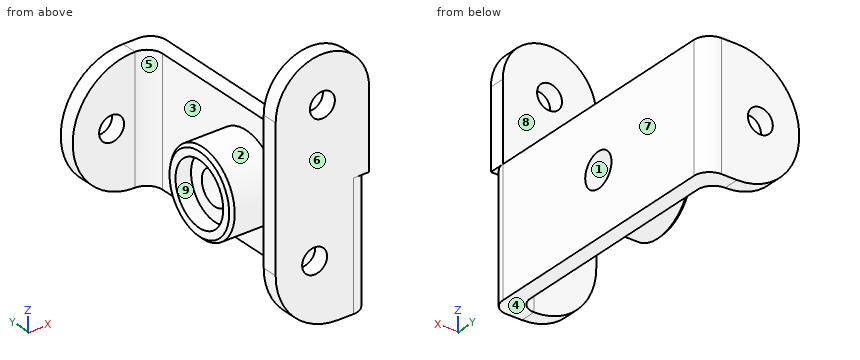
```python
from build123d import *

# Parameters (mm, degrees)
BOSS_EXTRUDE2_DEPTH             = 20
SKETCH2_R                       = 13.5
SKETCH2_R_2                     = 5.5
BOSS_EXTRUDE3_DEPTH             = 15
CUT_EXTRUDE1_DEPTH              = 56.226805086
CUT_EXTRUDE1_DEPTH_BACK         = 56.226805086
SKETCH2_3_R                     = 5.5
CHAMFER1_SIZE                   = 1
SKETCH3_R                       = 4
CUT_EXTRUDE2_DEPTH              = 10
FILLET2_RADIUS                  = 20
FILLET2_LENGTH                  = 5
FILLET3_RADIUS                  = 20
FILLET3_LENGTH                  = 5
SKETCH4_R                       = 4
CUT_EXTRUDE3_DEPTH              = 10
BOSS_EXTRUDE4_DEPTH             = 40
BOSS_EXTRUDE4_DIRECTION_2_REACH = 69.268
SKETCH7_R                       = 4
CUT_EXTRUDE4_DEPTH              = 30
FILLET5_RADIUS                  = 15
FILLET5_LENGTH                  = 5
SKETCH8_R                       = 10
CUT_EXTRUDE5_DEPTH              = 5


with BuildPart() as part:
    # Sketch1 → Boss-Extrude2 (new, symmetric)
    with BuildSketch(Plane.XY):
        with BuildLine():
            Line((0, 45), (25, 45))
            ThreePointArc((25, 45), (28.535533906, 43.535533906), (30, 40))
            Line((30, 40), (30, -40))
            ThreePointArc((30, -40), (28.535533906, -43.535533906), (25, -45))
            Line((25, -45), (0, -45))
            Line((0, -45), (0, -40))
            Line((0, -40), (20, -40))
            ThreePointArc((20, -40), (23.535533906, -38.535533906), (25, -35))
            Line((25, -35), (25, 35))
            ThreePointArc((25, 35), (23.535533906, 38.535533906), (20, 40))
            Line((20, 40), (0, 40))
            Line((0, 40), (0, 45))
        make_face()
    extrude(amount=BOSS_EXTRUDE2_DEPTH, both=True)

    # Sketch2 → Boss-Extrude3 (add)
    # profile 1 of 2: a face of its own
    with BuildSketch(Plane.ZY.offset(-25)):
        with Locations(Location((0, 0, 0), (0, 0, 180))):
            Circle(SKETCH2_R)
        Circle(SKETCH2_R_2, mode=Mode.SUBTRACT)
    # profile 2 of 2: a face of its own
    with BuildSketch(Plane.ZY.offset(-25)):
        Circle(SKETCH2_R_2)
    extrude(amount=BOSS_EXTRUDE3_DEPTH)

    # Sketch2<3> → Cut-Extrude1 (cut, two sides: drawn at the far end of the back side and taken through both)
    with BuildSketch(Plane.ZY.offset(-25).offset(-CUT_EXTRUDE1_DEPTH_BACK)):
        with Locations(Location((0, 0, 0), (0, 0, 270))):
            Circle(SKETCH2_3_R)
    extrude(amount=CUT_EXTRUDE1_DEPTH + CUT_EXTRUDE1_DEPTH_BACK, mode=Mode.SUBTRACT)

    # Chamfer1
    chamfer1_edges = [part.edges().sort_by_distance(p)[0] for p in [
        (10, 0, 13.5),
    ]]
    chamfer(chamfer1_edges, length=CHAMFER1_SIZE)

    # Sketch3 → Cut-Extrude2 (cut)
    with BuildSketch(Plane(origin=(0, 45, 0), x_dir=(1, 0, 0), z_dir=(0, 1, 0))):
        with Locations(Location((12.5, 0, 0), (0, 0, 180))):
            Circle(SKETCH3_R)
    extrude(amount=-CUT_EXTRUDE2_DEPTH, mode=Mode.SUBTRACT)

    # Fillet2: full round fillet: the end face becomes a half cylinder, R = half its width
    fillet2_face = Plane((0, 42.5, 0), x_dir=(0, -1, 0), z_dir=(-1, 0, 0))  # on the end face: x along it, z out of the body
    fillet2_slab = fillet2_face.offset(-FILLET2_RADIUS / 2) * Box(FILLET2_LENGTH, 2 * FILLET2_RADIUS, FILLET2_RADIUS, mode=Mode.PRIVATE)  # the body's end, R deep
    fillet2_round = Plane((20, 42.5, 0), x_dir=(-1, 0, 0), z_dir=(0, -1, 0)) * Cylinder(FILLET2_RADIUS, FILLET2_LENGTH, mode=Mode.PRIVATE)  # its axis R under the face
    add(fillet2_slab - fillet2_round, mode=Mode.SUBTRACT)

    # Fillet3: full round fillet: the end face becomes a half cylinder, R = half its width
    fillet3_face = Plane((0, -42.5, 0), x_dir=(0, -1, 0), z_dir=(-1, 0, 0))  # on the end face: x along it, z out of the body
    fillet3_slab = fillet3_face.offset(-FILLET3_RADIUS / 2) * Box(FILLET3_LENGTH, 2 * FILLET3_RADIUS, FILLET3_RADIUS, mode=Mode.PRIVATE)  # the body's end, R deep
    fillet3_round = Plane((20, -42.5, 0), x_dir=(-1, 0, 0), z_dir=(0, -1, 0)) * Cylinder(FILLET3_RADIUS, FILLET3_LENGTH, mode=Mode.PRIVATE)  # its axis R under the face
    add(fillet3_slab - fillet3_round, mode=Mode.SUBTRACT)

    # Sketch4 → Cut-Extrude3 (cut)
    with BuildSketch(Plane(origin=(0, -40, 0), x_dir=(1, 0, 0), z_dir=(0, 1, 0))):
        with Locations(Location((12.5, 0, 0), (0, 0, 180))):
            Circle(SKETCH4_R)
    extrude(amount=-CUT_EXTRUDE3_DEPTH, mode=Mode.SUBTRACT)

    # Sketch6 → Boss-Extrude4 (add)
    with BuildSketch(Plane.XY.offset(20)):
        Polygon((0, -40), (0, -45), (30, -45), (30, -40), (20, -40), align=None)
    extrude(amount=BOSS_EXTRUDE4_DEPTH)

    # Sketch6 → Boss-Extrude4 direction 2 (add, up to next)
    with BuildSketch(Plane.XY.offset(20), mode=Mode.PRIVATE) as boss_extrude4_direction_2_sk1:
        Polygon((0, -40), (0, -45), (30, -45), (30, -40), (20, -40), align=None)
    boss_extrude4_direction_2_tool1 = extrude(boss_extrude4_direction_2_sk1.sketch, amount=-BOSS_EXTRUDE4_DIRECTION_2_REACH, mode=Mode.PRIVATE) - part.part
    add(boss_extrude4_direction_2_tool1.solids().sort_by_distance((15, -42.5, 20))[0])

    # Sketch7 → Cut-Extrude4 (cut)
    with BuildSketch(Plane(origin=(0, -40, 0), x_dir=(1, 0, 0), z_dir=(0, 1, 0))):
        with Locations(Location((15, -45, 0), (0, 0, 180))):
            Circle(SKETCH7_R)
    extrude(amount=-CUT_EXTRUDE4_DEPTH, mode=Mode.SUBTRACT)

    # Fillet5: full round fillet: the end face becomes a half cylinder, R = half its width
    fillet5_face = Plane((15, -42.5, 60), x_dir=(0, -1, 0), z_dir=(0, 0, 1))  # on the end face: x along it, z out of the body
    fillet5_slab = fillet5_face.offset(-FILLET5_RADIUS / 2) * Box(FILLET5_LENGTH, 2 * FILLET5_RADIUS, FILLET5_RADIUS, mode=Mode.PRIVATE)  # the body's end, R deep
    fillet5_round = Plane((15, -42.5, 45), x_dir=(0, 0, 1), z_dir=(0, -1, 0)) * Cylinder(FILLET5_RADIUS, FILLET5_LENGTH, mode=Mode.PRIVATE)  # its axis R under the face
    add(fillet5_slab - fillet5_round, mode=Mode.SUBTRACT)

    # Sketch8 → Cut-Extrude5 (cut)
    with BuildSketch(Plane.ZY.offset(-10)):
        with Locations(Location((0, 0, 0), (0, 0, 270))):
            Circle(SKETCH8_R)
    extrude(amount=-CUT_EXTRUDE5_DEPTH, mode=Mode.SUBTRACT)


solid = part.part
```
Geometry: final body of the model. Coordinates: model frame, mm. Face numbers are marked on the shaded views. A direction names the side the tool comes from. Give positions to 0.01 mm unless a question says otherwise; leave off trailing zeros. Write each loop counter-clockwise with the first axis right and the second up, starting at its lowest first coordinate (ties: lowest second). Pieces come first, ordered by that corner, then holes.
1. Pin query (flat end, axial travel): P1, Ø1, axis at x = 8.5, z = 38.5, coming from the +Y side; P2, Ø14.5, axis at y = 0, z = 0, coming from the -X side; P3, Ø12, axis at x = 16, y = -23.5, coming from the +Z side; P4, Ø20, axis at y = -0.5, z = -1.5, coming from the -X side. Return the tip coordinate at first contact, or that it passes through.
2. Section query D-D, the plane x = 26. Return loops of the section in (y, z).
3. Section query C-C, the plane z = 47.5. Return loops of the section in (x, y).
4. Reachability of the marked faces 5, 6, 7, 8 and 9 from +Z, -Z, +X, -X, +Y, -Y: full face, straight path, thin tool, end or side. Return the list, or none.
5. Section query A-A, the plane y = 0. Return loops of the section in (x, z).
6. Line query: probe 1 along Y at (x, z) = (6, 13); probe 2 along Y at (x, z) = (19, 6); probe 3 along Z at (x, y) = (12.5, -42). Output: solid intervals per line, ascending.
7. Draft query along Z for the marked faces 1, 2, 3 and 4. Return one class per face: released by +Z, released by -Z, zero draft, split by the parting line, or undercut.
8. Section query B-B, the plane x = 12.5. Return loops of the section in (y, z).
Computed:
1. P1: stops at y = -40
1. P2: stops at x = 15
1. P3: passes through
1. P4: stops at x = 10
2. outline: (-45, 20) - (-44.9, 20) - (-44.9, -20) - (44.9, -20) - (44.9, 20) - (-40, 20) - (-40, 55.2) - (-45, 55.2) - close; hole circle Ø11 at (0, 0)
3. outline: (0.21, -45) - (11.88, -45) - (11.88, -40) - (0.21, -40) - close; (18.12, -45) - (29.79, -45) - (29.79, -40) - (18.12, -40) - close
4. face 5: +Z, -Z, -X
4. face 6: +Z, -Z, +X, -X, -Y
4. face 7: +Z, -Z, +X, +Y, -Y
4. face 8: +Z, -X
4. face 9: -X
5. outline: (10, -12.5) - (11, -13.5) - (25, -13.5) - (25, -20) - (30, -20) - (30, -5.5) - (15, -5.5) - (15, -10) - (10, -10) - close; (10, 10) - (15, 10) - (15, 5.5) - (30, 5.5) - (30, 20) - (25, 20) - (25, 13.5) - (11, 13.5) - (10, 12.5) - close
6. probe 1: y = -45 to -40, 40 to 45
6. probe 2: y = -45 to -40, -12.09 to 12.09, 40 to 45
6. probe 3: z = -18.54 to -4, 4 to 41.88, 48.12 to 59.79
7. face 1: undercut
7. face 2: split by the parting line
7. face 3: zero draft
7. face 4: released by -Z
8. outline: (-45, -18.54) - (-40, -18.54) - (-40, -4) - (-45, -4) - close; (-45, 4) - (-40, 4) - (-40, 41.88) - (-45, 41.88) - close; (-45, 48.12) - (-40, 48.12) - (-40, 59.79) - (-45, 59.79) - close; circle Ø27 at (0, 0); (40, -18.54) - (45, -18.54) - (45, -4) - (40, -4) - close; (40, 4) - (45, 4) - (45, 18.54) - (40, 18.54) - close; hole circle Ø20 at (0, 0)
